Could you check a few things on this model? Use its own coordinates, in mm. A direction names the side the tool comes from. Give positions to 0.01 mm unless a question says otherwise; leave off trailing zeros. Order: outer loops, then holes, each group sorted by start corner. A loop starts at its lowest first (then second) coordinate and runs counter-clockwise, first axis right, second up.
from build123d import *

# Parameters (mm, degrees)
F0_W     = 100
F0_H     = 100
F0_W_2   = 94
F0_H_2   = 94
F1_DEPTH = 1250
F2_R     = 5
F3_DEPTH = 300


with BuildPart() as f1:
    # F0 (on Top) → F1 (new body, symmetric)
    with BuildSketch(Plane.XY):
        Rectangle(F0_W, F0_H)
        Rectangle(F0_W_2, F0_H_2, mode=Mode.SUBTRACT)
    extrude(amount=F1_DEPTH, both=True)

    # F2 (on face) → F3 (cut)
    with BuildSketch(Plane.YZ.offset(50)):
        with Locations((0, 1200)):
            Circle(F2_R)
        with Locations((0, 700)):
            Circle(F2_R)
        with Locations((0, -700)):
            Circle(F2_R)
        with Locations((0, -1200)):
            Circle(F2_R)
    extrude(amount=-F3_DEPTH, mode=Mode.SUBTRACT)


solid = f1.part
Item 1: For faces 1 (the flat face through (47, -1, 18)), 2 (the flat face through (-1, -50, 18)), which set-ups out of +Z, -Z, +X, -X, +Y, -Y let a thin tool reach every point of the face, with its end or its side?
Findings:
face 1: +Z, -Z
face 2: +Z, -Z, +X, -X, -Y
Item 2: Please list where these lines run through material, in increasing order: line 1 along Z through (x, y) = (47.8, 0); line 2 along X through (y, z) = (-46, 900.5).
Findings:
line 1: z = -1250 to -1205, -1195 to -705, -695 to 695, 705 to 1195, 1205 to 1250
line 2: x = -50 to -47, 47 to 50
Item 3: Imagine slicing it at A-A on x = -6.5. List the corners of the cut face in (y, z) for me, then the cut area to 3 significant figures.
Findings:
outline: (-50, -1250) - (-47, -1250) - (-47, 1250) - (-50, 1250) - close; (47, -1250) - (50, -1250) - (50, 1250) - (47, 1250) - close
area: 15,000 mm2
Item 4: For pin 1 (13 mm diameter, centred on y = 0, z = -1200, fed in from -X), with a flat end and sliding along its axis, tell me the tip position at first contact or that it passes through.
Findings:
pin 1: stops at x = -50
Item 5: We'd pull the mould along X, two halves only. Please class faces 3 (the flat face through (-50, -1, 18)), 4 (the flat face through (-1, -47, 18)), 5 (the flat face through (50, -1, 18)): +X half, -X half, draft (parallel to the pull), parting line (faces both ways), or undercut.
Findings:
face 3: -X half
face 4: undercut
face 5: +X half
Item 6: Imagine slicing it at C-C on z = -609.5. List the corners of the cut face in (x, y) for me.
Findings:
outline: (-50, -50) - (50, -50) - (50, 50) - (-50, 50) - close; hole (-47, -47) - (47, -47) - (47, 47) - (-47, 47) - close
